Design review of the part built by this model. Coordinates are the model's own, in mm. Coordinates: 2 decimals unless noted, no trailing zeros. Loops run counter-clockwise (first coordinate to the right, second up) from the corner with the lowest first, then second, coordinate; pieces in that order, holes last. Notation, with made-up numbers: M 12,4.25 L 48,4.25 A27 cw 48,33.25 Z; hole C -7.5,-6.75 d7. An arc over 180 degrees is marked long. Put each result on its own line as item: value. Start each with the question number.
(1) The part is to be moulded in two halves that separate along X. For faces 1 (the cylindrical face through (28.803, 4.93, -20.319)), 2 (the cylindrical face through (25.816, 4.93, -18.503)), 3 (the flat face through (14, 10, 23)), say which applies: +X half, -X half, draft (parallel to the pull), parting line (faces both ways), or undercut.
(2) Clearance check with flat-ended pins moving along their axes: pin 1 (1.5 mm diameter, centred on x = 13, y = 1, fed in from +Z); pin 2 (5 mm diameter, centred on y = 8.5, z = 6, fed in from +X). State where each tip first meets the part, or that it passes through.
(3) Take a section at C-C, the plane y = 6.75. Give the boundary of the cut face in (x, z).
(4) For probe 1 along Z at (x, y) = (27, 8); probe 2 along Z at (x, y) = (-19, 6.25); probe 3 along Z at (x, y) = (-14.5, 3.5), list the stretches that pass through material, from the lowest coordinate up. Write a range as [from, to].
(5) Take a section at B-B, the plane z = 0. Give the boundary of the cut face in (x, y), then the cut area to 3 significant figures.
(6) Take a section at A-A, the plane x = 0. Give the boundary of the cut face in (y, z).
```python
from build123d import *

# Parameters (mm, degrees)
SKETCH_1_R      = 26.4
SKETCH_1_R_2    = 1.25
EXTRUDE_1_DEPTH = 10
FILLET_1_R      = 1


with BuildPart() as part:
    # 草图1 → 凸台-拉伸1 (new body)
    with BuildSketch(Plane(origin=(0, 0, 0), x_dir=(1, 0, 0), z_dir=(0, 1, 0))):
        with BuildLine():
            ThreePointArc((24.696486218, 19.391842834), (-25.619357757, -18.155123468), (26.480356643, 16.87455813))
            ThreePointArc((26.480356643, 16.87455813), (28.760584743, 20.381149753), (24.696486218, 19.391842834))
        make_face()
        with Locations(Location((0, 0, 0), (0, 0, 270))):
            Circle(SKETCH_1_R, mode=Mode.SUBTRACT)
        with Locations(Location((26.924802738, 19.080225301, 0), (0, 0, 270))):
            Circle(SKETCH_1_R_2, mode=Mode.SUBTRACT)
    extrude(amount=EXTRUDE_1_DEPTH)

    # 圆角1
    fillet_1_edges = [part.edges().sort_by_distance(p)[0] for p in [
        (0, 0, -26.4),
    ]]
    fillet(fillet_1_edges, radius=FILLET_1_R)


solid = part.part
```
Computed values:
1. face 1: undercut
1. face 2: undercut
1. face 3: draft
2. pin 1: stops at z = 28.91
2. pin 2: stops at x = 31.2
3. outline: M 24.7,-19.39 A2.25 ccw long 26.48,-16.87 A31.4 ccw long Z; hole C 0,0 d52.8; hole C 26.92,-19.08 d2.5
4. probe 1: z = [-21.33, -20.33], [-17.83, -16.83], [-16.03, 16.03]
4. probe 2: z = [-25, -18.33], [18.33, 25]
4. probe 3: z = [-27.85, -22.06], [22.06, 27.85]
5. outline: M -31.4,0 L -27.4,0 A1 ccw -26.4,1 L -26.4,10 L -31.4,10 Z; M 26.4,1 A1 ccw 27.4,0 L 31.4,0 L 31.4,10 L 26.4,10 Z
5. area: 99.6 mm^2
6. outline: M 0,-31.4 L 10,-31.4 L 10,-26.4 L 1,-26.4 A1 ccw 0,-27.4 Z; M 0,27.4 A1 ccw 1,26.4 L 10,26.4 L 10,31.4 L 0,31.4 Z
